Geometry check sheet. Reference: the model listing, model coordinates, mm. Face numbers are marked on the shaded views. A direction names the side the tool comes from. Round coordinates to 2 decimals unless told otherwise and drop trailing zeros. Order: outer loops, then holes, each group sorted by start corner. A loop starts at its lowest first (then second) coordinate and runs counter-clockwise, first axis right, second up.
(1) Cross-section at A-A on z = 0. Enter the section's corners in (x, y), and give its area (3 significant figures).
(2) Draft check along Z on the marked faces 1, 2 and 3. Enter one of: pulls with the +Z half, pulls with the -Z half, needs draft (parallel to the pull), parting line crosses it, or undercut.
(3) Gauge pin test, flat ends, axial feed: P1, Ø4, axis at x = -0.5, y = 5.5, coming from the +Z side; P2, Ø3, axis at x = 5.5, y = 0, coming from the -Z side; P3, Ø1, axis at y = 1.5, z = -5.5, coming from the +X side; P4, Ø5, axis at y = 0, z = 0, coming from the +X side. Record the tip position at first contact, or that the pin passes through.
(4) Cross-section at C-C on x = 6. Enter the section's corners in (y, z).
(5) Cross-section at D-D on x = -0.5. Enter the section's corners in (y, z).
(6) Set-up check for the marked faces 4 and 5: record each of +Z, -Z, +X, -X, +Y, -Y from which the full face is reachable in a straight line by a thin tool's end or side.
(7) Thickness scan on L1, parallel to Y at x = 0.5, z = 0; L2, parallel to X at y = 4, z = -4; L3, parallel to Y at x = 6, z = -4. Record the ranges inside material, lowest first.
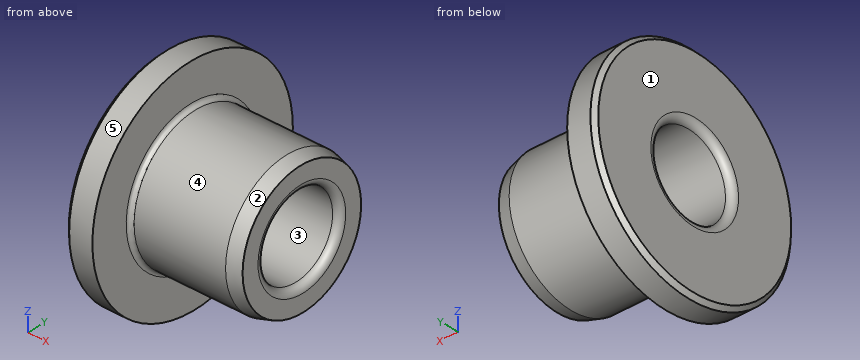
from build123d import *

# Parameters (mm, degrees)
CHAMFER1_SIZE = 0.3
FILLET1_R     = 0.3
FILLET5_R     = 0.5


with BuildPart() as part:
    # Sketch1 → Revolve1 (revolve)
    with BuildSketch(Plane.XY, mode=Mode.PRIVATE) as revolve1_sk:
        Polygon((-2, 3), (8, 3), (8, 5), (0, 5), (0, 8), (-2, 8), align=None)
    revolve(revolve1_sk.sketch.rotate(Axis((-2, 0, 0), (1, 0, 0)), 90), axis=Axis((-2, 0, 0), (1, 0, 0)))

    # Chamfer1
    chamfer1_edges = [part.edges().sort_by_distance(p)[0] for p in [
        (-2, 0, -8),
    ]]
    chamfer(chamfer1_edges, length=CHAMFER1_SIZE)

    # Fillet1
    fillet1_edges = [part.edges().sort_by_distance(p)[0] for p in [
        (0, 0, -5),
    ]]
    fillet(fillet1_edges, radius=FILLET1_R)

    # Chamfer3: read off the stored shape, not the designer's step
    # Chamfer3 outline → Chamfer3 (revolve, cut)
    with BuildSketch(Plane.YX):
        Polygon((5, 8), (4.732050808, 8), (5, 7), align=None)
    revolve(axis=Axis((0, 0, 0), (1, 0, 0)), mode=Mode.SUBTRACT)

    # Fillet5
    fillet5_edges = [part.edges().sort_by_distance(p)[0] for p in [
        (8, 0, -3),
        (-2, 0, -3),
    ]]
    fillet(fillet5_edges, radius=FILLET5_R)


solid = part.part
Found:
1. outline: (-2, -7.7) - (-1.7, -8) - (0, -8) - (0, -5.3) arc R0.3 cw to (0.3, -5) - (7, -5) - (8, -4.73) - (8, -3.5) arc R0.5 ccw to (7.5, -3) - (-1.5, -3) arc R0.5 ccw to (-2, -3.5) - close; (-2, 3.5) arc R0.5 ccw to (-1.5, 3) - (7.5, 3) arc R0.5 ccw to (8, 3.5) - (8, 4.73) - (7, 5) - (0.3, 5) arc R0.3 cw to (0, 5.3) - (0, 8) - (-1.7, 8) - (-2, 7.7) - close
1. area: 51.5 mm2
2. face 1: needs draft
2. face 2: parting line crosses it
2. face 3: undercut
3. P1: stops at z = 7.19
3. P2: stops at z = -5
3. P3: stops at x = 0.02
3. P4: passes through
4. outline: circle Ø10 at (0, 0); hole circle Ø6 at (0, 0)
5. outline: circle Ø16 at (0, 0); hole circle Ø6 at (0, 0)
6. face 4: +X
6. face 5: +X, -X
7. L1: y = -5 to -3, 3 to 5
7. L2: x = -2 to 0
7. L3: y = -3 to 3
